Input: part model. Units: mm. Frame: model coordinates. Coordinates: 2 decimals unless noted, no trailing zeros. Write each loop counter-clockwise with the first axis right and the second up, starting at its lowest first coordinate (ties: lowest second). Pieces come first, ordered by that corner, then holes. Notation, with made-up numbers: (63.5, 43) - (99.5, 43) arc R12 cw to (99.5, 63) - close; hole circle Ø10 at (-30, 89.25). An arc over 180 degrees is marked (long way). One line per question, with ' | ' between items. Start each with the question number.
1) Section query A-A on x = -24. Return loops of the section in (y, z), and give its area (3 significant figures).
2) Line query: line 1 (X direction, y = -46, z = -1.55); line 2 (Y direction, x = -57, z = -2.95); line 3 (Y direction, x = 20, z = -1.7). Output: solid intervals per line, ascending.
3) First-contact query: P1, Ø4, axis at x = -57, y = 46, coming from the +Z side. Flat tip, straight axial feed; report the tip coordinate or a pass-through.
4) Section query B-B on y = 26.5. Return loops of the section in (x, z).
5) Section query C-C on z = -1.5. Return loops of the section in (x, y).
```python
from build123d import *

# Parameters (mm, degrees)
SKETCH1_W           = 156
SKETCH1_H           = 106
BOSS_EXTRUDE1_DEPTH = 4
CUT_EXTRUDE1_REACH  = 96.387


with BuildPart() as part:
    # Sketch1 → Boss-Extrude1 (new body)
    with BuildSketch(Plane.XY):
        Rectangle(SKETCH1_W, SKETCH1_H)
    extrude(amount=-BOSS_EXTRUDE1_DEPTH)

    # Sketch2 → Cut-Extrude1 (cut, up to next)
    with BuildSketch(Plane.XY, mode=Mode.PRIVATE) as cut_extrude1_sk1:
        with BuildLine():
            ThreePointArc((60.25, 33.75), (59.373475383, 36.872498999), (57, 39.082682252))
            Line((57, 39.082682252), (57, -39.082682252))
            ThreePointArc((57, -39.082682252), (59.373475383, -36.872498999), (60.25, -33.75))
            Line((60.25, -33.75), (60.25, 33.75))
        make_face()
    cut_extrude1_tool1 = extrude(cut_extrude1_sk1.sketch, amount=-CUT_EXTRUDE1_REACH, mode=Mode.PRIVATE) & part.part
    # Sketch2 → Cut-Extrude1 (cut, up to next)
    with BuildSketch(Plane.XY, mode=Mode.PRIVATE) as cut_extrude1_sk2:
        with BuildLine():
            ThreePointArc((-54.25, 39.75), (-55.66490397, 39.580784403), (-57, 39.082682252))
            Line((-57, 39.082682252), (-57, -39.082682252))
            ThreePointArc((-57, -39.082682252), (-55.66490397, -39.580784403), (-54.25, -39.75))
            Line((-54.25, -39.75), (54.25, -39.75))
            ThreePointArc((54.25, -39.75), (55.66490397, -39.580784403), (57, -39.082682252))
            Line((57, -39.082682252), (57, 39.082682252))
            ThreePointArc((57, 39.082682252), (55.66490397, 39.580784403), (54.25, 39.75))
            Line((54.25, 39.75), (-54.25, 39.75))
        make_face()
    cut_extrude1_tool2 = extrude(cut_extrude1_sk2.sketch, amount=-CUT_EXTRUDE1_REACH, mode=Mode.PRIVATE) & part.part
    # Sketch2 → Cut-Extrude1 (cut, up to next)
    with BuildSketch(Plane.XY, mode=Mode.PRIVATE) as cut_extrude1_sk3:
        with BuildLine():
            Line((-57, -39.082682252), (-57, 39.082682252))
            ThreePointArc((-57, 39.082682252), (-59.373475383, 36.872498999), (-60.25, 33.75))
            Line((-60.25, 33.75), (-60.25, -33.75))
            ThreePointArc((-60.25, -33.75), (-59.373475383, -36.872498999), (-57, -39.082682252))
        make_face()
    cut_extrude1_tool3 = extrude(cut_extrude1_sk3.sketch, amount=-CUT_EXTRUDE1_REACH, mode=Mode.PRIVATE) & part.part
    # Sketch2 → Cut-Extrude1 (cut, up to next)
    with BuildSketch(Plane.XY, mode=Mode.PRIVATE) as cut_extrude1_sk4:
        with BuildLine():
            ThreePointArc((59.1, 46), (57, 48.1), (54.9, 46))
            Line((54.9, 46), (57, 46))
            Line((57, 46), (57, 43.9))
            ThreePointArc((57, 43.9), (58.48492424, 44.51507576), (59.1, 46))
        make_face()
    cut_extrude1_tool4 = extrude(cut_extrude1_sk4.sketch, amount=-CUT_EXTRUDE1_REACH, mode=Mode.PRIVATE) & part.part
    # Sketch2 → Cut-Extrude1 (cut, up to next)
    with BuildSketch(Plane.XY, mode=Mode.PRIVATE) as cut_extrude1_sk5:
        with BuildLine():
            Line((57, 46), (54.9, 46))
            ThreePointArc((54.9, 46), (55.51507576, 44.51507576), (57, 43.9))
            Line((57, 43.9), (57, 46))
        make_face()
    cut_extrude1_tool5 = extrude(cut_extrude1_sk5.sketch, amount=-CUT_EXTRUDE1_REACH, mode=Mode.PRIVATE) & part.part
    # Sketch2 → Cut-Extrude1 (cut, up to next)
    with BuildSketch(Plane.XY, mode=Mode.PRIVATE) as cut_extrude1_sk6:
        with BuildLine():
            ThreePointArc((59.1, 46), (57, 48.1), (54.9, 46))
            Line((54.9, 46), (57, 46))
            Line((57, 46), (57, 43.9))
            ThreePointArc((57, 43.9), (58.48492424, 44.51507576), (59.1, 46))
        make_face()
    cut_extrude1_tool6 = extrude(cut_extrude1_sk6.sketch, amount=-CUT_EXTRUDE1_REACH, mode=Mode.PRIVATE) & part.part
    # Sketch2 → Cut-Extrude1 (cut, up to next)
    with BuildSketch(Plane.XY, mode=Mode.PRIVATE) as cut_extrude1_sk7:
        with BuildLine():
            Line((57, 46), (54.9, 46))
            ThreePointArc((54.9, 46), (55.51507576, 44.51507576), (57, 43.9))
            Line((57, 43.9), (57, 46))
        make_face()
    cut_extrude1_tool7 = extrude(cut_extrude1_sk7.sketch, amount=-CUT_EXTRUDE1_REACH, mode=Mode.PRIVATE) & part.part
    # Sketch2 → Cut-Extrude1 (cut, up to next)
    with BuildSketch(Plane.XY, mode=Mode.PRIVATE) as cut_extrude1_sk8:
        with BuildLine():
            Line((-57, 43.9), (-57, 46))
            Line((-57, 46), (-54.9, 46))
            ThreePointArc((-54.9, 46), (-58.48492424, 47.48492424), (-57, 43.9))
        make_face()
    cut_extrude1_tool8 = extrude(cut_extrude1_sk8.sketch, amount=-CUT_EXTRUDE1_REACH, mode=Mode.PRIVATE) & part.part
    # Sketch2 → Cut-Extrude1 (cut, up to next)
    with BuildSketch(Plane.XY, mode=Mode.PRIVATE) as cut_extrude1_sk9:
        with BuildLine():
            Line((-54.9, 46), (-57, 46))
            Line((-57, 46), (-57, 43.9))
            ThreePointArc((-57, 43.9), (-55.51507576, 44.51507576), (-54.9, 46))
        make_face()
    cut_extrude1_tool9 = extrude(cut_extrude1_sk9.sketch, amount=-CUT_EXTRUDE1_REACH, mode=Mode.PRIVATE) & part.part
    # Sketch2 → Cut-Extrude1 (cut, up to next)
    with BuildSketch(Plane.XY, mode=Mode.PRIVATE) as cut_extrude1_sk10:
        with BuildLine():
            Line((-57, 43.9), (-57, 46))
            Line((-57, 46), (-54.9, 46))
            ThreePointArc((-54.9, 46), (-58.48492424, 47.48492424), (-57, 43.9))
        make_face()
    cut_extrude1_tool10 = extrude(cut_extrude1_sk10.sketch, amount=-CUT_EXTRUDE1_REACH, mode=Mode.PRIVATE) & part.part
    # Sketch2 → Cut-Extrude1 (cut, up to next)
    with BuildSketch(Plane.XY, mode=Mode.PRIVATE) as cut_extrude1_sk11:
        with BuildLine():
            Line((-54.9, 46), (-57, 46))
            Line((-57, 46), (-57, 43.9))
            ThreePointArc((-57, 43.9), (-55.51507576, 44.51507576), (-54.9, 46))
        make_face()
    cut_extrude1_tool11 = extrude(cut_extrude1_sk11.sketch, amount=-CUT_EXTRUDE1_REACH, mode=Mode.PRIVATE) & part.part
    # Sketch2 → Cut-Extrude1 (cut, up to next)
    with BuildSketch(Plane.XY, mode=Mode.PRIVATE) as cut_extrude1_sk12:
        with BuildLine():
            ThreePointArc((-54.9, -46), (-55.51507576, -44.51507576), (-57, -43.9))
            Line((-57, -43.9), (-57, -46))
            Line((-57, -46), (-54.9, -46))
        make_face()
    cut_extrude1_tool12 = extrude(cut_extrude1_sk12.sketch, amount=-CUT_EXTRUDE1_REACH, mode=Mode.PRIVATE) & part.part
    # Sketch2 → Cut-Extrude1 (cut, up to next)
    with BuildSketch(Plane.XY, mode=Mode.PRIVATE) as cut_extrude1_sk13:
        with BuildLine():
            Line((-57, -46), (-57, -43.9))
            ThreePointArc((-57, -43.9), (-58.48492424, -47.48492424), (-54.9, -46))
            Line((-54.9, -46), (-57, -46))
        make_face()
    cut_extrude1_tool13 = extrude(cut_extrude1_sk13.sketch, amount=-CUT_EXTRUDE1_REACH, mode=Mode.PRIVATE) & part.part
    # Sketch2 → Cut-Extrude1 (cut, up to next)
    with BuildSketch(Plane.XY, mode=Mode.PRIVATE) as cut_extrude1_sk14:
        with BuildLine():
            ThreePointArc((-54.9, -46), (-55.51507576, -44.51507576), (-57, -43.9))
            Line((-57, -43.9), (-57, -46))
            Line((-57, -46), (-54.9, -46))
        make_face()
    cut_extrude1_tool14 = extrude(cut_extrude1_sk14.sketch, amount=-CUT_EXTRUDE1_REACH, mode=Mode.PRIVATE) & part.part
    # Sketch2 → Cut-Extrude1 (cut, up to next)
    with BuildSketch(Plane.XY, mode=Mode.PRIVATE) as cut_extrude1_sk15:
        with BuildLine():
            Line((-57, -46), (-57, -43.9))
            ThreePointArc((-57, -43.9), (-58.48492424, -47.48492424), (-54.9, -46))
            Line((-54.9, -46), (-57, -46))
        make_face()
    cut_extrude1_tool15 = extrude(cut_extrude1_sk15.sketch, amount=-CUT_EXTRUDE1_REACH, mode=Mode.PRIVATE) & part.part
    # Sketch2 → Cut-Extrude1 (cut, up to next)
    with BuildSketch(Plane.XY, mode=Mode.PRIVATE) as cut_extrude1_sk16:
        with BuildLine():
            ThreePointArc((59.1, -46), (58.48492424, -44.51507576), (57, -43.9))
            Line((57, -43.9), (57, -46))
            Line((57, -46), (54.9, -46))
            ThreePointArc((54.9, -46), (57, -48.1), (59.1, -46))
        make_face()
    cut_extrude1_tool16 = extrude(cut_extrude1_sk16.sketch, amount=-CUT_EXTRUDE1_REACH, mode=Mode.PRIVATE) & part.part
    # Sketch2 → Cut-Extrude1 (cut, up to next)
    with BuildSketch(Plane.XY, mode=Mode.PRIVATE) as cut_extrude1_sk17:
        with BuildLine():
            Line((57, -46), (57, -43.9))
            ThreePointArc((57, -43.9), (55.51507576, -44.51507576), (54.9, -46))
            Line((54.9, -46), (57, -46))
        make_face()
    cut_extrude1_tool17 = extrude(cut_extrude1_sk17.sketch, amount=-CUT_EXTRUDE1_REACH, mode=Mode.PRIVATE) & part.part
    # Sketch2 → Cut-Extrude1 (cut, up to next)
    with BuildSketch(Plane.XY, mode=Mode.PRIVATE) as cut_extrude1_sk18:
        with BuildLine():
            ThreePointArc((59.1, -46), (58.48492424, -44.51507576), (57, -43.9))
            Line((57, -43.9), (57, -46))
            Line((57, -46), (54.9, -46))
            ThreePointArc((54.9, -46), (57, -48.1), (59.1, -46))
        make_face()
    cut_extrude1_tool18 = extrude(cut_extrude1_sk18.sketch, amount=-CUT_EXTRUDE1_REACH, mode=Mode.PRIVATE) & part.part
    # Sketch2 → Cut-Extrude1 (cut, up to next)
    with BuildSketch(Plane.XY, mode=Mode.PRIVATE) as cut_extrude1_sk19:
        with BuildLine():
            Line((57, -46), (57, -43.9))
            ThreePointArc((57, -43.9), (55.51507576, -44.51507576), (54.9, -46))
            Line((54.9, -46), (57, -46))
        make_face()
    cut_extrude1_tool19 = extrude(cut_extrude1_sk19.sketch, amount=-CUT_EXTRUDE1_REACH, mode=Mode.PRIVATE) & part.part
    add(cut_extrude1_tool1.solids().sort_by_distance((58.595694, 0, 0))[0], mode=Mode.SUBTRACT)
    add(cut_extrude1_tool2.solids().sort_by_distance((0, 0, 0))[0], mode=Mode.SUBTRACT)
    add(cut_extrude1_tool3.solids().sort_by_distance((-58.595694, 0, 0))[0], mode=Mode.SUBTRACT)
    add(cut_extrude1_tool4.solids().sort_by_distance((57.297089, 46.297089, 0))[0], mode=Mode.SUBTRACT)
    add(cut_extrude1_tool5.solids().sort_by_distance((56.108732, 45.108732, 0))[0], mode=Mode.SUBTRACT)
    add(cut_extrude1_tool6.solids().sort_by_distance((57.297089, 46.297089, 0))[0], mode=Mode.SUBTRACT)
    add(cut_extrude1_tool7.solids().sort_by_distance((56.108732, 45.108732, 0))[0], mode=Mode.SUBTRACT)
    add(cut_extrude1_tool8.solids().sort_by_distance((-57.297089, 46.297089, 0))[0], mode=Mode.SUBTRACT)
    add(cut_extrude1_tool9.solids().sort_by_distance((-56.108732, 45.108732, 0))[0], mode=Mode.SUBTRACT)
    add(cut_extrude1_tool10.solids().sort_by_distance((-57.297089, 46.297089, 0))[0], mode=Mode.SUBTRACT)
    add(cut_extrude1_tool11.solids().sort_by_distance((-56.108732, 45.108732, 0))[0], mode=Mode.SUBTRACT)
    add(cut_extrude1_tool12.solids().sort_by_distance((-56.108732, -45.108732, 0))[0], mode=Mode.SUBTRACT)
    add(cut_extrude1_tool13.solids().sort_by_distance((-57.297089, -46.297089, 0))[0], mode=Mode.SUBTRACT)
    add(cut_extrude1_tool14.solids().sort_by_distance((-56.108732, -45.108732, 0))[0], mode=Mode.SUBTRACT)
    add(cut_extrude1_tool15.solids().sort_by_distance((-57.297089, -46.297089, 0))[0], mode=Mode.SUBTRACT)
    add(cut_extrude1_tool16.solids().sort_by_distance((57.297089, -46.297089, 0))[0], mode=Mode.SUBTRACT)
    add(cut_extrude1_tool17.solids().sort_by_distance((56.108732, -45.108732, 0))[0], mode=Mode.SUBTRACT)
    add(cut_extrude1_tool18.solids().sort_by_distance((57.297089, -46.297089, 0))[0], mode=Mode.SUBTRACT)
    add(cut_extrude1_tool19.solids().sort_by_distance((56.108732, -45.108732, 0))[0], mode=Mode.SUBTRACT)


solid = part.part
```
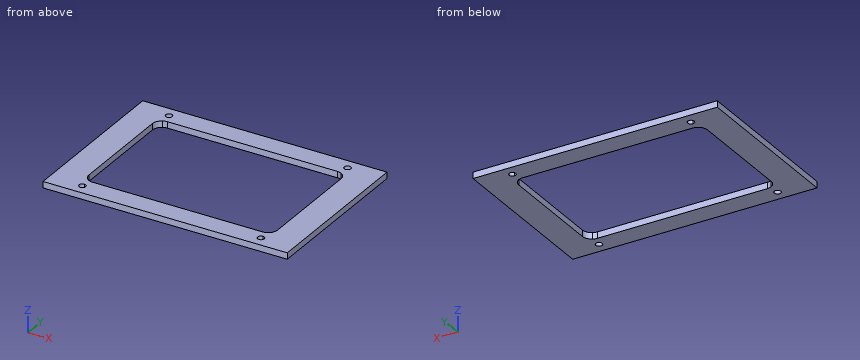
Answer key:
1) outline: (-53, -4) - (-39.75, -4) - (-39.75, 0) - (-53, 0) - close; (39.75, -4) - (53, -4) - (53, 0) - (39.75, 0) - close | area: 106 mm²
2) line 1: -78 to -59.1, -54.9 to 54.9, 59.1 to 78 | line 2: -53 to -48.1, -43.9 to -39.08, 39.08 to 43.9, 48.1 to 53 | line 3: -53 to -39.75, 39.75 to 53
3) P1: through
4) outline: (-78, -4) - (-60.25, -4) - (-60.25, 0) - (-78, 0) - close; (60.25, -4) - (78, -4) - (78, 0) - (60.25, 0) - close
5) outline: (-78, -53) - (78, -53) - (78, 53) - (-78, 53) - close; hole (-60.25, -33.75) arc R6 ccw to (-54.25, -39.75) - (54.25, -39.75) arc R6 ccw to (60.25, -33.75) - (60.25, 33.75) arc R6 ccw to (54.25, 39.75) - (-54.25, 39.75) arc R6 ccw to (-60.25, 33.75) - close; hole circle Ø4.2 at (-57, -46); hole circle Ø4.2 at (-57, 46); hole circle Ø4.2 at (57, -46); hole circle Ø4.2 at (57, 46)
